```python
from build123d import *

# Parameters (mm, degrees)
F1_DEPTH = 6.35
F2_SIZE  = 0.254


# Not quite as in the source:
# - a feature names something its author has since deleted; it is built from what else it names


with BuildPart() as f1:
    # F0 (on Front) → F1 (new body)
    with BuildSketch(Plane.XZ):
        with BuildLine():
            Line((0, 1.5875), (0, 15.875))
            ThreePointArc((0, 15.875), (0.79375, 16.66875), (1.5875, 15.875))
            Line((1.5875, 15.875), (1.5875, 3.175))
            Line((1.5875, 3.175), (3.175, 3.175))
            Line((3.175, 3.175), (3.175, 15.875))
            ThreePointArc((3.175, 15.875), (0.79375, 18.25625), (-1.5875, 15.875))
            Line((-1.5875, 15.875), (-1.5875, 2.749630657))
            ThreePointArc((-1.5875, 2.749630657), (-3.175, 0), (-1.5875, -2.749630657))
            Line((-1.5875, -2.749630657), (-1.5875, -14.2875))
            ThreePointArc((-1.5875, -14.2875), (0.79375, -16.66875), (3.175, -14.2875))
            Line((3.175, -14.2875), (3.175, -3.175))
            Line((3.175, -3.175), (1.5875, -3.175))
            Line((1.5875, -3.175), (1.5875, -14.2875))
            ThreePointArc((1.5875, -14.2875), (0.79375, -15.08125), (0, -14.2875))
            Line((0, -14.2875), (0, -1.5875))
            ThreePointArc((0, -1.5875), (-1.5875, 0), (0, 1.5875))
        make_face()
    extrude(amount=F1_DEPTH)

    # F2
    f2_edges = [f1.edges().sort_by_distance(p)[0] for p in [
        (-1.5875, -6.35, 9.312315),
        (0.79375, -6.35, 18.25625),
        (3.175, -6.35, 9.525),
        (-3.175, -6.35, 0),
        (-1.5875, -6.35, -8.518565),
        (0.79375, -6.35, -16.66875),
        (3.175, -6.35, -8.73125),
        (2.38125, -6.35, 3.175),
        (2.38125, -6.35, -3.175),
        (0, -6.35, -7.9375),
        (-1.5875, -6.35, 0),
        (0, -6.35, 8.73125),
        (1.5875, -3.175, 3.175),
        (1.5875, -3.175, -3.175),
        (2.38125, 0, -3.175),
        (3.175, -3.175, -3.175),
        (2.38125, 0, 3.175),
        (3.175, -3.175, 3.175),
        (3.175, 0, 9.525),
        (3.175, 0, -8.73125),
        (-3.175, 0, 0),
        (1.5875, 0, -8.73125),
        (1.5875, 0, 9.525),
        (-1.5875, 0, 0),
    ]]
    chamfer(f2_edges, length=F2_SIZE)


solid = f1.part
```
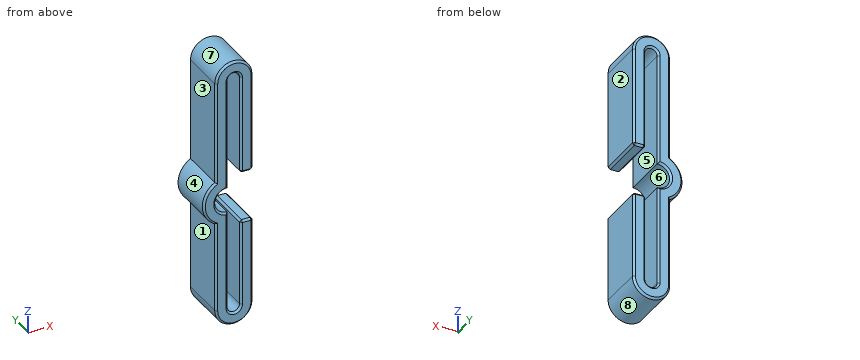
Geometry check sheet. Reference: the model listing, model coordinates, mm. Face numbers are marked on the shaded views. A direction names the side the tool comes from. Round coordinates to 2 decimals unless told otherwise and drop trailing zeros. Use a Markdown table: item, result. Add a question column.
1) Mould release check, pull along Z, two halves, no side actions. Record for the marked faces 6, 7 and 8: released by +Z, released by -Z, zero draft, split by the parting line, or undercut.
2) Thickness scan on line 1 along X through (y, z) = (-0.5, 10) (1 decimal); line 2 along Z through (x, y) = (0.75, -4); line 3 along Z through (x, y) = (2.5, -3.75) (3 decimals). Record the ranges inside material, lowest first.
3) Set-up check for the marked faces 1, 2, 3, 4 and 5: record each of +Z, -Z, +X, -X, +Y, -Y from which the full face is reachable in a straight line by a thin tool's end or side.
4) Gauge pin test, flat ends, axial feed: P1, Ø1.5, axis at x = 2, y = -3, coming from the -Z side; P2, Ø1.8, axis at y = -3, z = -7.5, coming from the -X side; P3, Ø1.2, axis at x = 2, y = -3.5, coming from the +Z side. Record the tip position at first contact, or that the pin passes through.
Established:
| question | item | result |
|---|---|---|
| 1 | face 6 | undercut |
| 1 | face 7 | released by +Z |
| 1 | face 8 | released by -Z |
| 2 | line 1 | -1.6 to 0, 1.6 to 3.2 |
| 2 | line 2 | -16.67 to -15.08, 16.67 to 18.26 |
| 2 | line 3 | -15.949 to -3.175, 3.175 to 17.536 |
| 3 | face 1 | -Z, -X, +Y, -Y |
| 3 | face 2 | +Z, -Z, +X, +Y, -Y |
| 3 | face 3 | +Z, -X, +Y, -Y |
| 3 | face 4 | -X, +Y, -Y |
| 3 | face 5 | +Y, -Y |
| 4 | P1 | z = -16.62 |
| 4 | P2 | x = -1.59 |
| 4 | P3 | z = 18.18 |
